Input: dimensioned drawing with shaded views. Units: mm. Origin: part minimum x, y, z. Round coordinates to 2 decimals unless told otherwise and drop trailing zeros. Write each loop counter-clockwise with the first axis right and the second up, starting at its lowest first coordinate (ties: lowest second). Pieces come first, ordered by that corner, then holes. Notation, with made-up numbers: (86, 76) -> (121, 76) arc R21 ccw to (121, 99) -> close; hole circle Ø9 at (6.25, 34). An arc over 180 degrees is marked (long way). Use one line per item in the form item = value. Start each with the question number.
1. Line query: L1, parallel to Y at x = 1.85, z = 57.5; L2, parallel to Z at x = 0.7, y = 2; L3, parallel to Y at x = 1.2, z = 4.5. Output: solid intervals per line, ascending.
2. Cut plane B-B, the plane z = 32.5. Return the cut outline in (x, y), plus the area to 3 significant figures.
3. Cut plane A-A, the plane y = 15. Return the cut outline in (x, z).
4. Cut plane C-C, the plane x = 1.35. State how many separate pieces and enclosed holes the cut face has, plus the area to 3 significant figures.
5. Cut plane D-D, the plane y = 27.25. Return the cut outline in (x, z), plus the area to 3 significant figures.
6. Pin query (flat end, axial travel): pin 1 Ø3 at (x, z) = (2.5, 28) entering from -Y; pin 2 Ø1.8 at (y, z) = (15, 32.5) entering from +X. Return the tip coordinate at first contact, or that it passes through.
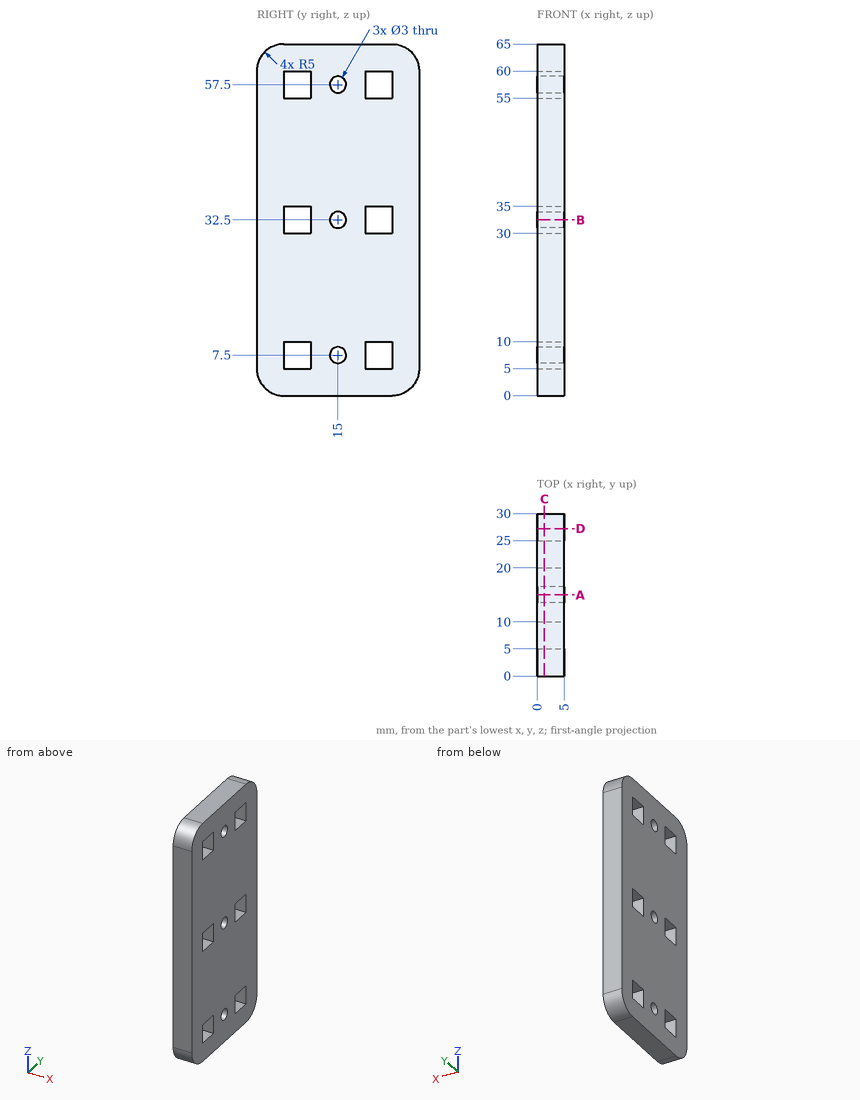
Outcome:
q1.L1 = 0 to 5, 10 to 13.5, 16.5 to 20, 25 to 30
q1.L2 = 1 to 64
q1.L3 = 0.03 to 29.97
q2.outline = (0, 0) -> (5, 0) -> (5, 5) -> (0, 5) -> close; (0, 10) -> (5, 10) -> (5, 13.5) -> (0, 13.5) -> close; (0, 16.5) -> (5, 16.5) -> (5, 20) -> (0, 20) -> close; (0, 25) -> (5, 25) -> (5, 30) -> (0, 30) -> close
q2.area = 85.0 mm^2
q3.outline = (0, 0) -> (5, 0) -> (5, 6) -> (0, 6) -> close; (0, 9) -> (5, 9) -> (5, 31) -> (0, 31) -> close; (0, 34) -> (5, 34) -> (5, 56) -> (0, 56) -> close; (0, 59) -> (5, 59) -> (5, 65) -> (0, 65) -> close
q4.separate_pieces = 1
q4.enclosed_holes = 9
q4.area = 1,760 mm^2
q5.outline = (0, 0.53) -> (5, 0.53) -> (5, 64.47) -> (0, 64.47) -> close
q5.area = 320 mm^2
q6.pin_1 = 0
q6.pin_2 = through
